Check sheet for the modelled part. Datum: model origin and axes. Units: mm. Round coordinates to 2 decimals unless told otherwise and drop trailing zeros. Order: outer loops, then holes, each group sorted by start corner. A loop starts at its lowest first (then second) coordinate and runs counter-clockwise, first axis right, second up.
```python
from build123d import *

# Parameters (mm, degrees)
CYLINDER029_R     = 2.1
CYLINDER029_DEPTH = 2
CYLINDER028_R     = 4
CYLINDER028_DEPTH = 2


with BuildPart() as cylinder029:
    # Cylinder029 → Cylinder029 (new body)
    with BuildSketch(Plane.XY):
        Circle(CYLINDER029_R)
    extrude(amount=CYLINDER029_DEPTH)


with BuildPart() as spacer:
    # Cylinder028 → Cylinder028 (new body)
    with BuildSketch(Plane.XY):
        Circle(CYLINDER028_R)
    extrude(amount=CYLINDER028_DEPTH)

    # Cut028006004005011004003001010002018: cut Cylinder029
    add(cylinder029.part, mode=Mode.SUBTRACT)


solid = spacer.part
```
Item 1: Sectioned sample at D-D (x = -3.25). Record the cut outline in (y, z).
Answer:
outline: (-2.33, 0) - (2.33, 0) - (2.33, 2) - (-2.33, 2) - close
Item 2: Sectioned sample at A-A (x = 0). Record the cut outline in (y, z), and give its area (3 significant figures).
Answer:
outline: (-4, 0) - (-2.1, 0) - (-2.1, 2) - (-4, 2) - close; (2.1, 0) - (4, 0) - (4, 2) - (2.1, 2) - close
area: 7.60 mm2
Item 3: Sectioned sample at C-C (z = 1.55). Record the cut outline in (x, y), and give its area (3 significant figures).
Answer:
outline: circle Ø8 at (0, 0); hole circle Ø4.2 at (0, 0)
area: 36.4 mm2
Item 4: Release check for a two-part mould opening along X. For faces 1 (the cylindrical face through (2.003, 0.631, 0.986)), 2 (the cylindrical face through (-0.867, -3.905, 0.986)), 3 (the flat face through (2, -2, 2)) record: released by +X, released by -X, zero draft, split by the parting line, or undercut.
Answer:
face 1: undercut
face 2: split by the parting line
face 3: zero draft
Item 5: Scan lines: line 1 along Y through (x, z) = (0, 0.8); line 2 along Y through (x, z) = (-0.5, 0.4); line 3 along X through (y, z) = (-1, 0.5). Record each from-to range of solid material in increasing order.
Answer:
line 1: y = -4 to -2.1, 2.1 to 4
line 2: y = -3.97 to -2.04, 2.04 to 3.97
line 3: x = -3.87 to -1.85, 1.85 to 3.87
